from build123d import *

# Parameters (mm, degrees)
BOSS_EXTRUDE1_DEPTH = 115
SKETCH3_W           = 20
SKETCH3_H           = 15
BOSS_EXTRUDE2_DEPTH = 1
SKETCH7_W           = 30
SKETCH7_H           = 15
BOSS_EXTRUDE5_DEPTH = 2


with BuildPart() as part:
    # Sketch2 → Boss-Extrude1 (new body)
    with BuildSketch(Plane(origin=(0, 0, 0), x_dir=(1, 0, 0), z_dir=(0, 1, 0))):
        Polygon((-10, 4.926686322), (-10, 0.926686322), (-7, 0.926686322), (-7, 2.926686322), (0, 2.926686322), (0, 3.926686322), (1, 3.926686322), (1, 2.926686322), (8, 2.926686322), (8, -8.073313678), (1, -8.073313678), (1, -9.073313678), (0, -9.073313678), (0, -8.073313678), (-7, -8.073313678), (-7, -6.073313678), (-10, -6.073313678), (-10, -10.073313678), (10, -10.073313678), (10, 4.926686322), align=None)
    extrude(amount=BOSS_EXTRUDE1_DEPTH)

    # Sketch3 → Boss-Extrude2 (add)
    with BuildSketch(Plane(origin=(0, 115, 0), x_dir=(1, 0, 0), z_dir=(0, 1, 0))):
        with Locations((0, -2.573313678)):
            Rectangle(SKETCH3_W, SKETCH3_H)
    extrude(amount=BOSS_EXTRUDE2_DEPTH)

    # Sketch7 → Boss-Extrude5 (add)
    with BuildSketch(Plane(origin=(0, 0, 0), x_dir=(-1, 0, 0), z_dir=(0, -1, 0))):
        with Locations((5, -2.573313678)):
            Rectangle(SKETCH7_W, SKETCH7_H)
    extrude(amount=BOSS_EXTRUDE5_DEPTH)


solid = part.part
Part model, mm, in its own coordinate system. A direction names the side the tool comes from. Give positions to 0.01 mm unless a question says otherwise; leave off trailing zeros. Loops run counter-clockwise (first coordinate to the right, second up) from the corner with the lowest first, then second, coordinate; pieces in that order, holes last. Notation, with made-up numbers: M 14.5,60 L 56.5,60 A19 ccw 56.5,83 Z; hole C 72.5,-18 d4. An arc over 180 degrees is marked long. Put each result on its own line as item: value. Start each with the question number.
1) Probe probe 1 along Y at (x, z) = (-8.5, 4.25); probe 2 along X at (y, z) = (54, 8.5); probe 3 along Z at (x, y) = (-2.5, 37). List the from-to ranges inside material, lowest first.
2) Saw through at D-D (x = -14.75). List the corners of the cut face in (y, z).
3) Pull direction Y, two halves, no side cores. Call faces 1 (the flat face through (-8, 57, 6.073)), 2 (the flat face through (-6, 0, 2)), 3 (the flat face through (0, 116, 2)), 4 (the flat face through (10, 58, 3)): +Y half, -Y half, draft (parallel to the pull), parting line (faces both ways), or undercut.
4) Flat gauge pins, fed straight in: pin 1 (3 mm diameter, centred on x = -13, z = 8, fed in from +Y); pin 2 (12 mm diameter, centred on x = -13, y = 45, fed in from -Z); pin 3 (0.8 mm diameter, centred on y = 41, z = 8.5, fed in from -X); pin 4 (1 mm diameter, centred on y = 91, z = 2, fed in from -X). Where does each tip first touch, or does it go through?
5) Saw through at C-C (y = 49). List the corners of the cut face in (x, z).
6) Saw through at B-B (z = 1.5). List the corners of the cut face in (x, y), then the cut area to 3 significant figures.
7) Saw through at A-A (x = -3.25). List the corners of the cut face in (y, z), then the cut area to 3 significant figures.
8) 3-axis set-ups, long thin cutter, end or side, ignore diameter. For faces 5 (the flat face through (-1, 58, -4.927)), 6 (the flat face through (-10, 57, -2)), 7 (the flat face through (-4, 57, -2.927)), 8 (the flat face through (-20, -1, 3)), 9 (the flat face through (-9, 57, -0.927)): which of +Z, -Z, +X, -X, +Y, -Y reach the whole face in a straight line?
Numbers:
1. probe 1: -2 to 0, 115 to 116
1. probe 2: -10 to 0, 1 to 10
1. probe 3: -4.93 to -2.93, 8.07 to 10.07
2. outline: M -2,-4.93 L 0,-4.93 L 0,10.07 L -2,10.07 Z
3. face 1: undercut
3. face 2: undercut
3. face 3: +Y half
3. face 4: draft
4. pin 1: y = 0
4. pin 2: z = -4.93
4. pin 3: x = -10
4. pin 4: x = 8
5. outline: M -10,-4.93 L 10,-4.93 L 10,10.07 L -10,10.07 L -10,6.07 L -7,6.07 L -7,8.07 L 0,8.07 L 0,9.07 L 1,9.07 L 1,8.07 L 8,8.07 L 8,-2.93 L 1,-2.93 L 1,-3.93 L 0,-3.93 L 0,-2.93 L -7,-2.93 L -7,-0.93 L -10,-0.93 Z
6. outline: M -20,-2 L 10,-2 L 10,116 L -10,116 L -10,115 L 8,115 L 8,0 L -20,0 Z
6. area: 310 mm^2
7. outline: M -2,-4.93 L 116,-4.93 L 116,10.07 L -2,10.07 Z; hole M 0,-2.93 L 115,-2.93 L 115,8.07 L 0,8.07 Z
7. area: 505 mm^2
8. face 5: -Z, +X, -X, +Y, -Y
8. face 6: +Z, -Z, -X, +Y
8. face 7: none
8. face 8: +Z, -Z, -X, +Y, -Y
8. face 9: -X
